Input: part model. Units: mm. Frame: model coordinates. A direction names the side the tool comes from. Give positions to 0.01 mm unless a question says otherwise; leave off trailing zeros. Write each loop counter-clockwise with the first axis right and the second up, starting at its lowest first coordinate (ties: lowest second). Pieces come first, ordered by that corner, then holes. Notation, with made-up numbers: (13, -28) -> (58, -28) arc R13 ccw to (58, -11) -> close; hole circle Ø8 at (11.5, 44). An arc over 180 degrees is marked (long way). Return JSON: item names as keys, results as strings. Group by question number.
Item 1: Line query: line 1 (X direction, y = 22, z = 18.5); line 2 (Y direction, x = 0, z = 1.3); line 3 (Y direction, x = 3.5, z = 9). Output: solid intervals per line, ascending. Write a range as [from, to].
Item 2: Mould query, pull axis X, two halves, no side actions, for faces 1 (the face through (0, 45, 10)), 2 (the face through (16.4, -44.43, 9.86)), 3 (the face through (10, -40.5, 18)). Classes: released by +X, released by -X, zero draft, split by the parting line, or undercut.
Item 3: Pin query (flat end, axial travel): P1, Ø6.5, axis at x = 2.5, y = -18, coming from the +Z side; P2, Ø4, axis at x = 1.5, z = 17.5, coming from the -Y side; P3, Ø5, axis at x = -1, y = -43.5, coming from the +Z side. Return the tip coordinate at first contact, or that it passes through.
Item 4: Section C-C, the plane z = 9.75. Return loops of the section in (x, y), then the cut area to 3 significant figures.
Item 5: Section A-A, the plane x = 0. Return loops of the section in (y, z), then the cut area to 3 significant figures.
Item 6: Set-up query: faces 4 (the face through (0, -42, 12.56)), 5 (the face through (-14, 7, 20)), 6 (the face through (0, -38.75, 8)). Return all of +Z, -Z, +X, -X, +Y, -Y with unobstructed straight access to the full face (end or side cutting, diameter ignored); none if empty.
Item 7: Section B-B, the plane y = 0. Return loops of the section in (x, z).
Item 8: Section D-D, the plane y = 37.5. Return loops of the section in (x, z), then the cut area to 3 significant figures.
from build123d import *

# Parameters (mm, degrees)
PAD_DEPTH       = 20
SKETCH001_W     = 26
SKETCH001_H     = 81
POCKET_DEPTH    = 3.5
SKETCH002_W     = 22
SKETCH002_H     = 77.5
POCKET001_DEPTH = 13.44
SKETCH003_W     = 14.5
SKETCH003_H     = 7.44
POCKET002_DEPTH = 45
SKETCH004_R     = 5
POCKET003_DEPTH = 3.061


with BuildPart() as part:
    # Sketch → Pad (new body)
    with BuildSketch(Plane.XY):
        with BuildLine():
            Line((-17, 43), (-17, -43))
            ThreePointArc((-17, -43), (-16.414214, -44.414214), (-15, -45))
            Line((-15, -45), (15, -45))
            ThreePointArc((15, -45), (16.414214, -44.414214), (17, -43))
            Line((17, -43), (17, 43))
            ThreePointArc((17, 43), (16.414214, 44.414214), (15, 45))
            Line((15, 45), (-15, 45))
            ThreePointArc((-15, 45), (-16.414214, 44.414214), (-17, 43))
        make_face()
    extrude(amount=PAD_DEPTH)

    # Sketch001 (on Face10 of Pad) → Pocket (cut)
    with BuildSketch(Plane.XY.offset(20)):
        Rectangle(SKETCH001_W, SKETCH001_H)
    extrude(amount=-POCKET_DEPTH, mode=Mode.SUBTRACT)

    # Sketch002 (on Face15 of Pocket) → Pocket001 (cut)
    with BuildSketch(Plane.XY.offset(16.5)):
        Rectangle(SKETCH002_W, SKETCH002_H)
    extrude(amount=-POCKET001_DEPTH, mode=Mode.SUBTRACT)

    # Sketch003 (on Face7 of Pocket001) → Pocket002 (cut)
    with BuildSketch(Plane.XZ.offset(45)):
        with Locations((0, 16.28)):
            Rectangle(SKETCH003_W, SKETCH003_H)
    extrude(amount=-POCKET002_DEPTH, mode=Mode.SUBTRACT)

    # Sketch004 (on Face24 of Pocket002) → Pocket003 (cut, through all)
    with BuildSketch(Plane.XY.offset(3.06)):
        Circle(SKETCH004_R)
    extrude(amount=-POCKET003_DEPTH, mode=Mode.SUBTRACT)


solid = part.part
Answer below:
{
 "1": {"line 1": "x = [-17, -13], [13, 17]", "line 2": "y = [-45, -5], [5, 45]", "line 3": "y = [-45, -38.75], [38.75, 45]"},
 "2": {"face 1": "zero draft", "face 2": "released by +X", "face 3": "undercut"},
 "3": {"P1": "stops at z = 3.06", "P2": "stops at y = 38.75", "P3": "stops at z = 12.56"},
 "4": {"outline": "(-17, -43) arc R2 ccw to (-15, -45) -> (15, -45) arc R2 ccw to (17, -43) -> (17, 43) arc R2 ccw to (15, 45) -> (-15, 45) arc R2 ccw to (-17, 43) -> close; hole (-11, -38.75) -> (11, -38.75) -> (11, 38.75) -> (-11, 38.75) -> close", "area": "1,350 mm2"},
 "5": {"outline": "(-45, 0) -> (-5, 0) -> (-5, 3.06) -> (-38.75, 3.06) -> (-38.75, 12.56) -> (-45, 12.56) -> close; (5, 0) -> (45, 0) -> (45, 20) -> (40.5, 20) -> (40.5, 16.5) -> (38.75, 16.5) -> (38.75, 3.06) -> (5, 3.06) -> close", "area": "404 mm2"},
 "6": {"face 4": "+Z, -Y", "face 5": "+Z, +X, -X, +Y, -Y", "face 6": "+Z"},
 "7": {"outline": "(-17, 0) -> (-5, 0) -> (-5, 3.06) -> (-11, 3.06) -> (-11, 16.5) -> (-13, 16.5) -> (-13, 20) -> (-17, 20) -> close; (5, 0) -> (17, 0) -> (17, 20) -> (13, 20) -> (13, 16.5) -> (11, 16.5) -> (11, 3.06) -> (5, 3.06) -> close"},
 "8": {"outline": "(-17, 0) -> (17, 0) -> (17, 20) -> (13, 20) -> (13, 16.5) -> (11, 16.5) -> (11, 3.06) -> (-11, 3.06) -> (-11, 16.5) -> (-13, 16.5) -> (-13, 20) -> (-17, 20) -> close", "area": "293 mm2"}
}
